Build history of the part. All positions in model axes, mm. A direction names the side the tool comes from. Give positions to 0.01 mm unless a question says otherwise; leave off trailing zeros. Order: outer loops, then holes, each group sorted by start corner. A loop starts at its lowest first (then second) coordinate and runs counter-clockwise, first axis right, second up. Notation, with made-up numbers: (1.5, -20) -> (51.5, -20) arc R15 cw to (51.5, -14) -> close; hole circle Ø1 at (36, 19). An arc over 180 degrees is marked (long way). Use a Markdown table: item, result. Add a question column.
```python
from build123d import *

# Parameters (mm, degrees)
SKETCH_2_R      = 3
EXTRUDE_1_DEPTH = 20
CHAMFER_1_SIZE  = 0.5


with BuildPart() as part:
    # ｽｹｯﾁ2 → ﾎﾞｽ - 押し出し1 (new, symmetric)
    with BuildSketch(Plane.XY):
        Circle(SKETCH_2_R)
    extrude(amount=EXTRUDE_1_DEPTH, both=True)

    # ｽｹｯﾁ4 → M3 ねじ穴1 (revolve, cut)
    with BuildSketch(Plane(origin=(0, 0, 20), x_dir=(0, -1, 0), z_dir=(1, 0, 0))):
        Polygon((0, 0), (0, 9.251075774), (1.25, 8.5), (1.25, 0), align=None)
    hole_wizard_m3_1 = revolve(axis=Axis((0, 0, 26.35), (0, 0, -1)), mode=Mode.SUBTRACT)

    # ﾐﾗｰ1: M3 ねじ穴1 across plane
    add(hole_wizard_m3_1.mirror(Plane.XY), mode=Mode.SUBTRACT)

    # 面取り1
    chamfer_1_edges = [part.edges().sort_by_distance(p)[0] for p in [
        (-3, 0, -20),
        (-3, 0, 20),
    ]]
    chamfer(chamfer_1_edges, length=CHAMFER_1_SIZE)


solid = part.part
```
(1) Band-saw the part on B-B on z = -0.5. Give the cut face in (x, y), plus the area to 3 significant figures.
(2) Pin check, flat tips, straight feed: pin 1 Ø1.5 at (x, y) = (0, 0) entering from +Z; pin 2 Ø2 at (y, z) = (0.5, 5) entering from +X; pin 3 Ø1 at (x, z) = (-1, -9) entering from +Y; pin 4 Ø2 at (x, y) = (0, 0) entering from +Z. Stop position of each tip, or through.
(3) Mould opens along Y. For faces 1 (the face through (1.22, 0.27, 15.81)), 2 (the face through (-3, 0, 0)), 3 (the face through (1, 1, -20)) say: released by +Y, released by -Y, zero draft, split by the parting line, or undercut.
(4) Band-saw the part on A-A on z = -17. Give the cut face in (x, y).
(5) Wall check: probe 1 along Y at (x, z) = (0, 18); probe 2 along Y at (x, z) = (-0.8, 18.5); probe 3 along X at (y, z) = (-0.5, -15). Give the ranges that are in metal, low to high.
(6) Tool access for faces 4 (the face through (1, 1, 20)), 5 (the face through (1.22, 0.27, -15.81)): list every direction of +Z, -Z, +X, -X, +Y, -Y with a clear straight run to the whole face (end or side of a thin tool).
Response:
| question | item | result |
|---|---|---|
| 1 | outline | circle Ø6 at (0, 0) |
| 1 | area | 28.3 mm² |
| 2 | pin 1 | stops at z = 11.2 |
| 2 | pin 2 | stops at x = 3 |
| 2 | pin 3 | stops at y = 2.96 |
| 2 | pin 4 | stops at z = 11.35 |
| 3 | face 1 | undercut |
| 3 | face 2 | split by the parting line |
| 3 | face 3 | zero draft |
| 4 | outline | circle Ø6 at (0, 0); hole circle Ø2.5 at (0, 0) |
| 5 | probe 1 | y = -3 to -1.25, 1.25 to 3 |
| 5 | probe 2 | y = -2.89 to -0.96, 0.96 to 2.89 |
| 5 | probe 3 | x = -2.96 to -1.15, 1.15 to 2.96 |
| 6 | face 4 | +Z, +X, -X, +Y, -Y |
| 6 | face 5 | -Z |
